from build123d import *

# Parameters (mm, degrees)
ESBO_O1_R                 = 12.5
RESSALTO_EXTRUS_O1_DEPTH  = 20
CORTE_EXTRUS_O3_DEPTH     = 11
ESBO_O3_R                 = 3.175
CORTE_EXTRUS_O4_DEPTH     = 21
ESBO_O6_W                 = 12
ESBO_O6_H                 = 2
CORTE_EXTRUS_O5_DEPTH     = 10
CORTE_EXTRUS_O6_START     = -3
ESBO_O7_R                 = 3.25
CORTE_EXTRUS_O6_DEPTH     = 9.5
FURO_ROSCADO_DE_M3X0_51_D = 2.5
FILETE1_R                 = 1
ESBO_O10_R                = 1.5
CORTE_EXTRUS_O7_DEPTH     = 1
CHANFRO1_SIZE             = 0.5
CORTE_EXTRUS_O8_REACH     = 18.5
ESBO_O11_R                = 1.5
ESBO_O12_R                = 6
CORTE_EXTRUS_O9_DEPTH     = 11
PADR_OCIRCULAR1_COUNT     = 4
CHANFRO2_SIZE             = 0.5


with BuildPart() as part:
    # Esboço1 → Ressalto-extrusão1 (new body)
    with BuildSketch(Plane.XY):
        Circle(ESBO_O1_R)
    extrude(amount=RESSALTO_EXTRUS_O1_DEPTH)

    # Esboço2 → Corte-extrusão3 (cut)
    with BuildSketch(Plane.XY.offset(20)):
        with BuildLine():
            Line((0, 0), (6.25, 10.825317547))
            ThreePointArc((6.25, 10.825317547), (12.5, 0), (6.25, -10.825317547))
            Line((6.25, -10.825317547), (0, 0))
        make_face()
    corte_extrus_o3 = extrude(amount=-CORTE_EXTRUS_O3_DEPTH, mode=Mode.SUBTRACT)

    # Esboço3 → Corte-extrusão4 (cut, through all)
    with BuildSketch(Plane(origin=(0, 0, 0), x_dir=(-1, 0, 0), z_dir=(0, 0, -1))):
        Circle(ESBO_O3_R)
    extrude(amount=-CORTE_EXTRUS_O4_DEPTH, mode=Mode.SUBTRACT)

    # Espelhar1: Corte-extrusão3 across plane
    add(corte_extrus_o3.mirror(Plane(origin=(0, 0, 0), x_dir=(0, 0, 1), z_dir=(1, 0, 0))), mode=Mode.SUBTRACT)

    # Esboço6 → Corte-extrusão5 (cut, through all)
    with BuildSketch(Plane.XY.offset(9)):
        with Locations((7, 0)):
            Rectangle(ESBO_O6_W, ESBO_O6_H)
    extrude(amount=-CORTE_EXTRUS_O5_DEPTH, mode=Mode.SUBTRACT)

    # Esboço7 → Corte-extrusão6 (cut, through all)
    with BuildSketch(Plane.XZ.offset(-1).offset(CORTE_EXTRUS_O6_START)):
        with Locations((8.459935794, 4.5)):
            Circle(ESBO_O7_R)
    extrude(amount=-CORTE_EXTRUS_O6_DEPTH, mode=Mode.SUBTRACT)

    # Furo roscado de M3x0.51 (through all)
    with Locations(Plane(origin=(0, 4, 0), x_dir=(1, 0, 0), z_dir=(0, 1, 0))):
        with Locations((8.459935794, -4.5)):
            Hole(FURO_ROSCADO_DE_M3X0_51_D / 2)

    # Filete1
    filete1_edges = [part.edges().sort_by_distance(p)[0] for p in [
        (-12.5, 0, 0),
    ]]
    fillet(filete1_edges, radius=FILETE1_R)

    # Esboço10 → Corte-extrusão7 (cut)
    with BuildSketch(Plane.XY.offset(9)):
        with Locations((6.363961031, -6.363961031)):
            Circle(ESBO_O10_R)
    corte_extrus_o7 = extrude(amount=-CORTE_EXTRUS_O7_DEPTH, mode=Mode.SUBTRACT)

    # Chanfro1
    chanfro1_edges = [part.edges().sort_by_distance(p)[0] for p in [
        (0, -12.5, 20),
        (0, 12.5, 20),
    ]]
    chamfer(chanfro1_edges, length=CHANFRO1_SIZE)

    # Esboço11 → Corte-extrusão8 (cut, up to next)
    with BuildSketch(Plane(origin=(0, 4, 0), x_dir=(1, 0, 0), z_dir=(0, 1, 0)), mode=Mode.PRIVATE) as corte_extrus_o8_sk1:
        with Locations((8.459935794, -4.5)):
            Circle(ESBO_O11_R)
    corte_extrus_o8_tool1 = extrude(corte_extrus_o8_sk1.sketch, amount=-CORTE_EXTRUS_O8_REACH, mode=Mode.PRIVATE) & part.part
    add(corte_extrus_o8_tool1.solids().sort_by_distance((8.459936, 4, 4.5))[0], mode=Mode.SUBTRACT)

    # Esboço12 → Corte-extrusão9 (cut)
    with BuildSketch(Plane.XY.offset(20)):
        Circle(ESBO_O12_R)
    extrude(amount=-CORTE_EXTRUS_O9_DEPTH, mode=Mode.SUBTRACT)

    # PadrãoCircular1: Corte-extrusão7 ×4 about axis
    padr_ocircular1_axis = Axis((0, 0, 0), (0, 0, 1))
    for i in range(1, PADR_OCIRCULAR1_COUNT):
        add(corte_extrus_o7.rotate(padr_ocircular1_axis, i * 360 / PADR_OCIRCULAR1_COUNT), mode=Mode.SUBTRACT)

    # Chanfro2
    chanfro2_edges = [part.edges().sort_by_distance(p)[0] for p in [
        (-3.175, 0, 0),
    ]]
    chamfer(chanfro2_edges, length=CHANFRO2_SIZE)


solid = part.part
Geometry: final body of the model. Coordinates: model frame, mm. A direction names the side the tool comes from. Give positions to 0.01 mm unless a question says otherwise; leave off trailing zeros. Order: outer loops, then holes, each group sorted by start corner. A loop starts at its lowest first (then second) coordinate and runs counter-clockwise, first axis right, second up. Notation, with made-up numbers: (23.5, 51) -> (80.5, 51) arc R17 cw to (80.5, 79) -> close; hole circle Ø7 at (-38.5, 89.25). An arc over 180 degrees is marked (long way). Answer as a JSON object with one key per item and string values.
Q1. Section D-D (y = 0). Output: boundary loops of the cut face in (x, z) (3 decimals), plus the area to 3 significant figures.
Entries:
{"outline": "(-12.5, 1) arc R1 ccw to (-11.5, 0) -> (-3.675, 0) -> (-3.175, 0.5) -> (-3.175, 9) -> (-12.5, 9) -> close", "area": "83.6 mm^2"}
Q2. Section B-B (x = 0). Output: boundary loops of the cut face in (y, z) (3 decimals), plus the area to 3 significant figures.
Entries:
{"outline": "(-12.5, 1) arc R1 ccw to (-11.5, 0) -> (-3.675, 0) -> (-3.175, 0.5) -> (-3.175, 9) -> (-6, 9) -> (-6, 20) -> (-12, 20) -> (-12.5, 19.5) -> close; (3.175, 0.5) -> (3.675, 0) -> (11.5, 0) arc R1 ccw to (12.5, 1) -> (12.5, 19.5) -> (12, 20) -> (6, 20) -> (6, 9) -> (3.175, 9) -> close", "area": "310 mm^2"}
Q3. Material intervals for probe 1 along X at (y, z) = (1.5, 4.25); probe 2 along Y at (x, z) = (3.5, 13); probe 3 along Y at (x, z) = (2, 13), sorted ascending.
Entries:
{"probe 1": "x = -12.41 to -2.8, 2.8 to 6.98, 9.94 to 12.41", "probe 2": "y = -12 to -6.06, 6.06 to 12", "probe 3": "y = -12.34 to -5.66, 5.66 to 12.34"}
Q4. Section A-A (z = 14). Output: boundary loops of the cut face in (x, y), plus the area to 3 significant figures.
Entries:
{"outline": "(-6.25, -10.83) arc R12.5 ccw to (6.25, -10.83) -> (3, -5.2) arc R6 cw to (-3, -5.2) -> close; (-6.25, 10.83) -> (-3, 5.2) arc R6 cw to (3, 5.2) -> (6.25, 10.83) arc R12.5 ccw to start", "area": "126 mm^2"}
Q5. Section C-C (z = 4.5). State how many separate pieces and enclosed holes the cut face has, plus the area to 3 significant figures.
Entries:
{"separate pieces": "3", "enclosed holes": "0", "area": "380 mm^2"}
Q6. Access query for faces 5 (the flat face through (4.6, 7.97, 14.58)), 6 (the flat face through (6.6, 1, 4.6)), 7 (the cylindrical face through (7.75, -6.94, 8.51)), 8 (the flat face through (-4.648, -8.05, 14.577)). Directions: +Z, -Z, +X, -X, +Y, -Y. A direction counts if a zero-diameter tool reaches every point of the face in a straight line with its end or side. Return the directions, or none.
Entries:
{"face 5": "+Z, +X", "face 6": "+Z, -Z, +X", "face 7": "+Z", "face 8": "+Z, -X"}
Q7. First-contact query: pin 1 (10.5 mm diameter, centred on x = 8.46, z = 4.5, fed in from +Y); pin 2 (7 mm diameter, centred on x = 6.5, z = 4, fed in from -Y); pin 3 (3 mm diameter, centred on x = -5.5, z = 8, fed in from +Y). Flat tips, straight axial feed; report the tip coordinate or a pass-through.
Entries:
{"pin 1": "stops at y = 12.08", "pin 2": "stops at y = -12.13", "pin 3": "stops at y = 11.84"}
Q8. Draft query along Z for faces 1 (the cylindrical face through (6.96, 2.52, 4.43)), 2 (the cylindrical face through (5.213, 6.812, 4.643)), 3 (the cylindrical face through (6.94, 7.75, 8.51)), 4 (the flat face through (0, -9, 20)). Return one class per face: released by +Z, released by -Z, zero draft, split by the parting line, or undercut.
Entries:
{"face 1": "undercut", "face 2": "undercut", "face 3": "zero draft", "face 4": "released by +Z"}
